```python
from build123d import *

# Parameters (mm, degrees)
EXTRUDE_1_DEPTH      = 32.5
CUT_EXTRUDE_3_DEPTH  = 30.5
EXTRUDE_2_DEPTH      = 68
CUT_EXTRUDE_8_DEPTH  = 69
SKETCH_11_R          = 19.1
SKETCH_11_R_2        = 2.6
CUT_EXTRUDE_10_DEPTH = 69
CHAMFER_1_SIZE       = 6
CHAMFER_2_SIZE       = 6
CHAMFER_3_SIZE       = 6
CHAMFER_4_SIZE       = 6
FILLET_1_R           = 2


with BuildPart() as part:
    # 草图1 → 凸台-拉伸1 (new body, symmetric)
    with BuildSketch(Plane(origin=(0, 0, 0), x_dir=(0, 0, -1), z_dir=(1, 0, 0))):
        Polygon((-68, 0), (0, 0), (0, 68), (-2, 68), (-2, 27), (-17, 2), (-68, 2), align=None)
    extrude(amount=EXTRUDE_1_DEPTH, both=True)

    # 草图6 → 切除-拉伸3 (cut, symmetric)
    with BuildSketch(Plane(origin=(0, 0, 0), x_dir=(0, 0, -1), z_dir=(1, 0, 0))):
        Polygon((-17, 2), (-2, 27), (-2, 2), align=None)
    extrude(amount=CUT_EXTRUDE_3_DEPTH, both=True, mode=Mode.SUBTRACT)

    # 草图7 → 凸台-拉伸2 (add, through all)
    with BuildSketch(Plane(origin=(0, 0, 0), x_dir=(1, 0, 0), z_dir=(0, 1, 0))):
        with BuildLine():
            Line((-17.9, -16), (-17.9, -58))
            ThreePointArc((-17.9, -58), (-20, -60.1), (-22.1, -58))
            Line((-22.1, -58), (-22.1, -16))
            ThreePointArc((-22.1, -16), (-20, -13.9), (-17.9, -16))
        make_face()
        with BuildLine():
            Line((17.9, -16), (17.9, -58))
            ThreePointArc((17.9, -58), (20, -60.1), (22.1, -58))
            Line((22.1, -58), (22.1, -16))
            ThreePointArc((22.1, -16), (20, -13.9), (17.9, -16))
        make_face()
    extrude(amount=EXTRUDE_2_DEPTH)

    # 草图10 → 切除-拉伸8 (cut, through all)
    with BuildSketch(Plane(origin=(0, 0, 0), x_dir=(1, 0, 0), z_dir=(0, 1, 0))):
        with BuildLine():
            Line((-17.9, -16), (-17.9, -58))
            ThreePointArc((-17.9, -58), (-20, -60.1), (-22.1, -58))
            Line((-22.1, -58), (-22.1, -16))
            ThreePointArc((-22.1, -16), (-20, -13.9), (-17.9, -16))
        make_face()
        with BuildLine():
            Line((17.9, -16), (17.9, -58))
            ThreePointArc((17.9, -58), (20, -60.1), (22.1, -58))
            Line((22.1, -58), (22.1, -16))
            ThreePointArc((22.1, -16), (20, -13.9), (17.9, -16))
        make_face()
    extrude(amount=CUT_EXTRUDE_8_DEPTH, mode=Mode.SUBTRACT)

    # 草图11 → 切除-拉伸10 (cut, through all)
    with BuildSketch(Plane.XY):
        with Locations((0, 39)):
            Circle(SKETCH_11_R)
        with Locations((-23.5, 62.5)):
            Circle(SKETCH_11_R_2)
        with Locations((23.5, 62.5)):
            Circle(SKETCH_11_R_2)
        with Locations((23.5, 15.5)):
            Circle(SKETCH_11_R_2)
        with Locations((-23.5, 15.5)):
            Circle(SKETCH_11_R_2)
    extrude(amount=CUT_EXTRUDE_10_DEPTH, mode=Mode.SUBTRACT)

    # 倒角1
    chamfer_1_edges = [part.edges().sort_by_distance(p)[0] for p in [
        (-32.5, 68, 1),
    ]]
    chamfer(chamfer_1_edges, length=CHAMFER_1_SIZE)

    # 倒角2
    chamfer_2_edges = [part.edges().sort_by_distance(p)[0] for p in [
        (32.5, 68, 1),
    ]]
    chamfer(chamfer_2_edges, length=CHAMFER_2_SIZE)

    # 倒角3
    chamfer_3_edges = [part.edges().sort_by_distance(p)[0] for p in [
        (-32.5, 1, 68),
    ]]
    chamfer(chamfer_3_edges, length=CHAMFER_3_SIZE)

    # 倒角4
    chamfer_4_edges = [part.edges().sort_by_distance(p)[0] for p in [
        (32.5, 1, 68),
    ]]
    chamfer(chamfer_4_edges, length=CHAMFER_4_SIZE)

    # 圆角1
    fillet_1_edges = [part.edges().sort_by_distance(p)[0] for p in [
        (0, 0, 0),
    ]]
    fillet(fillet_1_edges, radius=FILLET_1_R)


solid = part.part
```
Geometry: final body of the model. Coordinates: model frame, mm. A direction names the side the tool comes from. Coordinates: 2 decimals unless noted, no trailing zeros. Loops run counter-clockwise (first coordinate to the right, second up) from the corner with the lowest first, then second, coordinate; pieces in that order, holes last. Notation, with made-up numbers: (32.5, 85.5) -> (59.5, 85.5) arc R18 cw to (59.5, 120.5) -> close; hole circle Ø11 at (2, -0.75). An arc over 180 degrees is marked (long way). Use a Markdown table: item, result. Add a question column.
(1) Section query D-D, the plane x = 0. Return loops of the section in (y, z).
(2) Section query A-A, the plane z = 37.5. Return loops of the section in (x, y), plus the area to 3 significant figures.
(3) Access query for faces 4 (the cylindrical face through (25.9, 14.5, 1)), 5 (the flat face through (-22.1, 1, 37)), 6 (the flat face through (0, 2, 35)). Directions: +Z, -Z, +X, -X, +Y, -Y. A direction counts if a zero-diameter tool reaches every point of the face in a straight line with its end or side. Return the directions, or none.
(4) Section query B-B, the plane x = 23.5. Return loops of the section in (y, z), plus the area to 3 significant figures.
(5) Section query C-C, the plane y = 15.5. Return loops of the section in (x, z).
(6) Line query: line 1 along X through (y, z) = (10, 10); line 2 along Y through (x, z) = (23.5, 1.4); line 3 along Y through (x, z) = (-23, 1). Output: solid intervals per line, ascending.
(7) Mould query, pull axis Y, two halves, no side actions, for faces 1 (the flat face through (0, 0, 35)), 2 (the cylindrical face through (-21.1, 14.5, 1)), 3 (the flat face through (-7, 20, 0)). Classes: pulls with the +Y half, pulls with the -Y half, needs draft (parallel to the pull), parting line crosses it, or undercut.
(8) Pin query (flat end, axial travel): pin 1 Ø6 at (x, z) = (14.5, 34) entering from +Y; pin 2 Ø3 at (x, y) = (23.5, 15.5) entering from +Z; pin 3 Ø8 at (x, y) = (-0.5, 61) entering from -Z; pin 4 Ø7 at (x, y) = (-23.5, 15.5) entering from +Z. Return the tip coordinate at first contact, or that it passes through.
Answer:
| question | item | result |
|---|---|---|
| 1 | outline | (0, 2) arc R2 ccw to (2, 0) -> (19.9, 0) -> (19.9, 2) -> (2, 2) -> (2, 68) -> (0, 68) -> close; (58.1, 0) -> (68, 0) -> (68, 2) -> (58.1, 2) -> close |
| 2 | outline | (-32.5, 0) -> (-22.1, 0) -> (-22.1, 2) -> (-32.5, 2) -> close; (-17.9, 0) -> (17.9, 0) -> (17.9, 2) -> (-17.9, 2) -> close; (22.1, 0) -> (32.5, 0) -> (32.5, 2) -> (22.1, 2) -> close |
| 2 | area | 113 mm^2 |
| 3 | face 4 | +Z, -Z |
| 3 | face 5 | +Y, -Y |
| 3 | face 6 | +Z, +Y |
| 4 | outline | (0, 2) arc R2 ccw to (2, 0) -> (12.9, 0) -> (12.9, 2) -> (2, 2) -> (2, 68) -> (0, 68) -> close; (18.1, 0) -> (59.9, 0) -> (59.9, 2) -> (18.1, 2) -> close; (65.1, 0) -> (68, 0) -> (68, 2) -> (65.1, 2) -> close |
| 4 | area | 246 mm^2 |
| 5 | outline | (-32.5, 0) -> (-26.1, 0) -> (-26.1, 2) -> (-30.5, 2) -> (-30.5, 8.9) -> (-32.5, 8.9) -> close; (-20.9, 0) -> (20.9, 0) -> (20.9, 2) -> (-20.9, 2) -> close; (26.1, 0) -> (32.5, 0) -> (32.5, 8.9) -> (30.5, 8.9) -> (30.5, 2) -> (26.1, 2) -> close |
| 6 | line 1 | x = -32.5 to -30.5, 30.5 to 32.5 |
| 6 | line 2 | y = 0.09 to 12.9, 18.1 to 59.9, 65.1 to 68 |
| 6 | line 3 | y = 0.27 to 12.95, 18.05 to 59.95, 65.05 to 68 |
| 7 | face 1 | pulls with the -Y half |
| 7 | face 2 | undercut |
| 7 | face 3 | needs draft |
| 8 | pin 1 | stops at y = 2 |
| 8 | pin 2 | passes through |
| 8 | pin 3 | stops at z = 0 |
| 8 | pin 4 | stops at z = 2 |
